from build123d import *

# Parameters (mm, degrees)
SKETCH_1_W          = 36
SKETCH_1_H          = 36
SKETCH_1_R          = 7.5
EXTRUDE_1_DEPTH     = 11
EXTRUDE_START       = 11
SKETCH_1_3_R        = 7.5
EXTRUDE_2_DEPTH     = 9
SKETCH_2_R          = 2
CUT_EXTRUDE_1_DEPTH = 3
CUT_EXTRUDE_START   = -33
SKETCH_2_2_R        = 2
CUT_EXTRUDE_2_DEPTH = 3


with BuildPart() as part:
    # 草图1 → 凸台-拉伸1 (new body)
    # profile 1 of 2: a face of its own
    with BuildSketch(Plane.XY):
        with Locations((18, 18)):
            Rectangle(SKETCH_1_W, SKETCH_1_H)
        with Locations((18, 18)):
            Circle(SKETCH_1_R, mode=Mode.SUBTRACT)
    # profile 2 of 2: a face of its own
    with BuildSketch(Plane.XY):
        with Locations((18, 18)):
            Circle(SKETCH_1_R)
    extrude(amount=EXTRUDE_1_DEPTH)

    # 草图1<3> → 凸台-拉伸2 (add)
    with BuildSketch(Plane.XY.offset(EXTRUDE_START)):
        with Locations((18, 18)):
            Circle(SKETCH_1_3_R)
    extrude(amount=EXTRUDE_2_DEPTH)

    # 草图2 → 切除-拉伸1 (cut)
    with BuildSketch(Plane(origin=(36, 0, 0), x_dir=(0, 0, -1), z_dir=(1, 0, 0))):
        with Locations((-5.5, 18)):
            Circle(SKETCH_2_R)
    extrude(amount=-CUT_EXTRUDE_1_DEPTH, mode=Mode.SUBTRACT)

    # 草图2<2> → 切除-拉伸2 (cut)
    with BuildSketch(Plane(origin=(36, 0, 0), x_dir=(0, 0, -1), z_dir=(1, 0, 0)).offset(CUT_EXTRUDE_START)):
        with Locations((-5.5, 18)):
            Circle(SKETCH_2_2_R)
    extrude(amount=-CUT_EXTRUDE_2_DEPTH, mode=Mode.SUBTRACT)


solid = part.part
Geometry: final body of the model. Coordinates: model frame, mm. A direction names the side the tool comes from. Round coordinates to 2 decimals unless told otherwise and drop trailing zeros. Loops run counter-clockwise (first coordinate to the right, second up) from the corner with the lowest first, then second, coordinate; pieces in that order, holes last. Notation, with made-up numbers: (14, 39) -> (63, 39) arc R19 cw to (63, 46) -> close; hole circle Ø5 at (66.25, 22). An arc over 180 degrees is marked (long way). One line per question, with ' | ' between items. Start each with the question number.
1. Section A-A on z = 5.5. Output: boundary loops of the cut face in (x, y).
2. Set-up query: faces 1 (the face through (18, 10, 11)), 2 (the face through (1.521, 19.983, 5.76)), 3 (the face through (18, 36, 5)). Return all of +Z, -Z, +X, -X, +Y, -Y with unobstructed straight access to the full face (end or side cutting, diameter ignored); none if empty.
3. Contact query for flat-ended pins moving along their axis: pin 1 (3 mm diameter, centred on y = 18, z = 4.5, fed in from +X); pin 2 (3.5 mm diameter, centred on y = 18, z = 5.5, fed in from +X); pin 3 (3.5 mm diameter, centred on y = 18, z = 5.5, fed in from -X); pin 4 (4 mm diameter, centred on x = 9.5, z = 16, fed in from -Y). Output: stop coordinate, or through.
4. Section B-B on x = 18. Output: boundary loops of the cut face in (y, z), and give its area (3 significant figures).
5. Section D-D on x = 11.5. Output: boundary loops of the cut face in (y, z).
6. Section C-C on y = 18. Output: boundary loops of the cut face in (x, z), and give its area (3 significant figures).
7. Line query: line 1 along Y through (x, z) = (1, 5.5); line 2 along Z through (x, y) = (31.5, 4); line 3 along Y through (x, z) = (20, 19). Output: solid intervals per line, ascending. Write a range as [from, to].
8. Mould query, pull axis Y, two halves, no side actions, for faces 4 (the face through (12.5, 23.1, 15.4)), 5 (the face through (0, 18, 3)), 6 (the face through (33, 18, 6)), 7 (the face through (34.521, 19.983, 5.76)). Classes: pulls with the +Y half, pulls with the -Y half, needs draft (parallel to the pull), parting line crosses it, or undercut.
Returned:
1) outline: (0, 0) -> (36, 0) -> (36, 16) -> (33, 16) -> (33, 20) -> (36, 20) -> (36, 36) -> (0, 36) -> (0, 20) -> (3, 20) -> (3, 16) -> (0, 16) -> close
2) face 1: +Z | face 2: -X | face 3: +Z, -Z, +X, -X, +Y
3) pin 1: stops at x = 36 | pin 2: stops at x = 33 | pin 3: stops at x = 3 | pin 4: stops at y = 14.26
4) outline: (0, 0) -> (36, 0) -> (36, 11) -> (25.5, 11) -> (25.5, 20) -> (10.5, 20) -> (10.5, 11) -> (0, 11) -> close | area: 531 mm2
5) outline: (0, 0) -> (36, 0) -> (36, 11) -> (21.74, 11) -> (21.74, 20) -> (14.26, 20) -> (14.26, 11) -> (0, 11) -> close
6) outline: (0, 0) -> (36, 0) -> (36, 3.5) -> (33, 3.5) -> (33, 7.5) -> (36, 7.5) -> (36, 11) -> (25.5, 11) -> (25.5, 20) -> (10.5, 20) -> (10.5, 11) -> (0, 11) -> (0, 7.5) -> (3, 7.5) -> (3, 3.5) -> (0, 3.5) -> close | area: 507 mm2
7) line 1: y = [0, 16], [20, 36] | line 2: z = [0, 11] | line 3: y = [10.77, 25.23]
8) face 4: parting line crosses it | face 5: needs draft | face 6: undercut | face 7: undercut
